from build123d import *

# Parameters (mm, degrees)
SKETCH1_W               = 96
SKETCH1_H               = 76
BOSS_EXTRUDE1_DEPTH     = 1.5
SKETCH2_W               = 6
SKETCH2_H               = 2
SKETCH2_W_2             = 2
SKETCH2_H_2             = 6
BOSS_EXTRUDE2_DEPTH     = 4
CUT_EXTRUDE1_REACH      = 63.351
SKETCH3_R               = 1.5
MIRROR2_COPY_1_REACH    = 63.351
MIRROR2_COPY_1_SKETCH_R = 1.5


with BuildPart() as part:
    # Sketch1 → Boss-Extrude1 (new body)
    with BuildSketch(Plane(origin=(0, 0, 0), x_dir=(1, 0, 0), z_dir=(0, 1, 0))):
        Rectangle(SKETCH1_W, SKETCH1_H)
    extrude(amount=BOSS_EXTRUDE1_DEPTH)

    # Sketch2 → Boss-Extrude2 (add)
    with BuildSketch(Plane(origin=(0, 1.5, 0), x_dir=(1, 0, 0), z_dir=(0, 1, 0))):
        with Locations((0, 34.9)):
            Rectangle(SKETCH2_W, SKETCH2_H)
        with Locations((-44.9, 0)):
            Rectangle(SKETCH2_W_2, SKETCH2_H_2)
        with Locations((0, -34.9)):
            Rectangle(SKETCH2_W, SKETCH2_H)
        with Locations((44.9, 0)):
            Rectangle(SKETCH2_W_2, SKETCH2_H_2)
    extrude(amount=BOSS_EXTRUDE2_DEPTH)

    # Sketch3 → Cut-Extrude1 (cut, up to next)
    with BuildSketch(Plane(origin=(0, 1.5, 0), x_dir=(1, 0, 0), z_dir=(0, 1, 0)), mode=Mode.PRIVATE) as cut_extrude1_sk1:
        with Locations(Location((-41, -31, 0), (0, 0, 270))):
            Circle(SKETCH3_R)
    cut_extrude1_tool1 = extrude(cut_extrude1_sk1.sketch, amount=-CUT_EXTRUDE1_REACH, mode=Mode.PRIVATE) & part.part
    cut_extrude1 = cut_extrude1_tool1.solids().sort_by_distance((-41, 1.5, 31))[0]
    add(cut_extrude1, mode=Mode.SUBTRACT)

    # Mirror1: Cut-Extrude1 across plane
    add(cut_extrude1.mirror(Plane.XY), mode=Mode.SUBTRACT)

    # Mirror2: Cut-Extrude1 across plane
    add(cut_extrude1.mirror(Plane(origin=(0, 0, 0), x_dir=(0, 0, 1), z_dir=(1, 0, 0))), mode=Mode.SUBTRACT)

    # Mirror2 copy 1 sketch → Mirror2 copy 1 (cut, up to next)
    with BuildSketch(Plane(origin=(0, 1.5, 0), x_dir=(-1, 0, 0), z_dir=(0, 1, 0)), mode=Mode.PRIVATE) as mirror2_copy_1_sk1:
        with Locations(Location((-41, -31, 0), (0, 0, 270))):
            Circle(MIRROR2_COPY_1_SKETCH_R)
    mirror2_copy_1_tool1 = extrude(mirror2_copy_1_sk1.sketch, amount=-MIRROR2_COPY_1_REACH, mode=Mode.PRIVATE) & part.part
    add(mirror2_copy_1_tool1.solids().sort_by_distance((41, 1.5, -31))[0], mode=Mode.SUBTRACT)


solid = part.part
Check sheet for the modelled part. Datum: model origin and axes. Units: mm. A direction names the side the tool comes from. Round coordinates to 2 decimals unless told otherwise and drop trailing zeros. Loops run counter-clockwise (first coordinate to the right, second up) from the corner with the lowest first, then second, coordinate; pieces in that order, holes last. Notation, with made-up numbers: (19.5, 70.25) -> (64.5, 70.25) arc R18 cw to (64.5, 81.25) -> close; hole circle Ø8 at (32, 82.25). An arc over 180 degrees is marked (long way). Put each result on its own line as item: value. Start each with the question number.
1. Section check C-C (z = 31). Enter the section's corners in (x, y).
2. Scan lines: probe 1 along X at (y, z) = (0.85, 31); probe 2 along Z at (x, y) = (41, 1.05); probe 3 along Y at (x, z) = (21.5, 28). Record each from-to range of solid material in increasing order.
3. Draft check along Z on faces 4 (the face through (45.9, 3, 0)), 5 (the face through (0, 3, 33.9)), 6 (the face through (0, 3, -35.9)). Enter one of: +Z half, -Z half, draft (parallel to the pull), parting line (faces both ways), or undercut.
4. Gauge pin test, flat ends, axial feed: pin 1 (2.5 mm diameter, centred on x = 41, z = 31, fed in from +Y); pin 2 (4 mm diameter, centred on x = 41, z = -31, fed in from +Y); pin 3 (2 mm diameter, centred on x = 1.5, y = 4.5, fed in from +Z); pin 4 (1.6 mm diameter, centred on y = 4, z = 35.5, fed in from +X). Record the tip position at first contact, or that the pin passes through.
5. Section check A-A (y = 3.9). Enter the section's corners in (x, z), plus the area to 3 significant figures.
6. Access from +Z, -Z, +X, -X, +Y, -Y to the whole of each face (thin tool, end or side, straight path). Record for faces 1 (the face through (0, 3, -33.9)), 2 (the face through (-45.9, 3, 0)), 3 (the face through (43.9, 3, 0)).
7. Section check D-D (x = -2). Enter the section's corners in (y, z).
8. Section check B-B (x = 41). Enter the section's corners in (y, z), plus the area to 3 significant figures.
Findings:
1. outline: (-48, 0) -> (-42.5, 0) -> (-42.5, 1.5) -> (-48, 1.5) -> close; (-39.5, 0) -> (39.5, 0) -> (39.5, 1.5) -> (-39.5, 1.5) -> close; (42.5, 0) -> (48, 0) -> (48, 1.5) -> (42.5, 1.5) -> close
2. probe 1: x = -48 to -42.5, -39.5 to 39.5, 42.5 to 48
2. probe 2: z = -38 to -32.5, -29.5 to 29.5, 32.5 to 38
2. probe 3: y = 0 to 1.5
3. face 4: draft
3. face 5: undercut
3. face 6: -Z half
4. pin 1: passes through
4. pin 2: stops at y = 1.5
4. pin 3: stops at z = 35.9
4. pin 4: stops at x = 3
5. outline: (-45.9, -3) -> (-43.9, -3) -> (-43.9, 3) -> (-45.9, 3) -> close; (-3, -35.9) -> (3, -35.9) -> (3, -33.9) -> (-3, -33.9) -> close; (-3, 33.9) -> (3, 33.9) -> (3, 35.9) -> (-3, 35.9) -> close; (43.9, -3) -> (45.9, -3) -> (45.9, 3) -> (43.9, 3) -> close
5. area: 48.0 mm^2
6. face 1: +X, -X, +Y
6. face 2: +Z, -Z, -X, +Y
6. face 3: +Z, -Z, +Y
7. outline: (0, -38) -> (1.5, -38) -> (1.5, -35.9) -> (5.5, -35.9) -> (5.5, -33.9) -> (1.5, -33.9) -> (1.5, 33.9) -> (5.5, 33.9) -> (5.5, 35.9) -> (1.5, 35.9) -> (1.5, 38) -> (0, 38) -> close
8. outline: (0, -38) -> (1.5, -38) -> (1.5, -32.5) -> (0, -32.5) -> close; (0, -29.5) -> (1.5, -29.5) -> (1.5, 29.5) -> (0, 29.5) -> close; (0, 32.5) -> (1.5, 32.5) -> (1.5, 38) -> (0, 38) -> close
8. area: 105 mm^2
